The listing builds one solid part. Answer for the finished solid, in the listing's coordinates (mm). A direction names the side the tool comes from. Give positions to 0.01 mm unless a question says otherwise; leave off trailing zeros. Write each loop counter-clockwise with the first axis right and the second up, starting at its lowest first coordinate (ties: lowest second). Pieces come first, ordered by that corner, then holes. Notation, with made-up numbers: (-13, -0.5) - (40, -0.5) arc R18 cw to (40, 24.5) - close; hole circle Ø11 at (22, -3.5). An arc over 180 degrees is marked (long way). One line per item, written item: value. Start each with the question number.
from build123d import *

# Parameters (mm, degrees)
SKETCH_1_W      = 50
SKETCH_1_H      = 14
SKETCH_1_R      = 3
EXTRUDE_1_DEPTH = 5
SKETCH_2_W      = 35
SKETCH_2_H      = 14
EXTRUDE_2_DEPTH = 15
SKETCH_3_W      = 35
SKETCH_3_H      = 5
EXTRUDE_3_DEPTH = 8
SKETCH_4_W      = 12
SKETCH_4_H      = 4
SKETCH_4_W_2    = 6
EXTRUDE_4_DEPTH = 4
FILLET_1_R      = 2


with BuildPart() as part:
    # Эскиз1 → Бобышка-Вытянуть1 (new body)
    with BuildSketch(Plane(origin=(0, 0, 0), x_dir=(1, 0, 0), z_dir=(0, 1, 0))):
        with Locations((-18, 0)):
            Rectangle(SKETCH_1_W, SKETCH_1_H)
        with Locations(Location((0, 0, 0), (0, 0, 270))):
            Circle(SKETCH_1_R, mode=Mode.SUBTRACT)
    extrude(amount=EXTRUDE_1_DEPTH)

    # Эскиз2 → Бобышка-Вытянуть2 (add)
    with BuildSketch(Plane(origin=(0, 5, 0), x_dir=(1, 0, 0), z_dir=(0, 1, 0))):
        with Locations((-25.5, 0)):
            Rectangle(SKETCH_2_W, SKETCH_2_H)
    extrude(amount=EXTRUDE_2_DEPTH)

    # Эскиз3 → Бобышка-Вытянуть3 (add)
    with BuildSketch(Plane(origin=(0, 20, 0), x_dir=(1, 0, 0), z_dir=(0, 1, 0))):
        with Locations((-25.5, -4.5)):
            Rectangle(SKETCH_3_W, SKETCH_3_H)
        with Locations((-25.5, 4.5)):
            Rectangle(SKETCH_3_W, SKETCH_3_H)
    extrude(amount=EXTRUDE_3_DEPTH)

    # Эскиз4 → Бобышка-Вытянуть4 (add)
    with BuildSketch(Plane(origin=(0, 20, 0), x_dir=(1, 0, 0), z_dir=(0, 1, 0))):
        with Locations((-49, 0)):
            Rectangle(SKETCH_4_W, SKETCH_4_H)
        with Locations((-5, 0)):
            Rectangle(SKETCH_4_W_2, SKETCH_4_H)
    extrude(amount=-EXTRUDE_4_DEPTH)

    # Скругление1
    fillet_1_edges = [part.edges().sort_by_distance(p)[0] for p in [
        (-25.5, 28, 7),
        (-25.5, 28, 2),
        (-25.5, 28, -7),
        (-25.5, 28, -2),
    ]]
    fillet(fillet_1_edges, radius=FILLET_1_R)


solid = part.part
Item 1: Each of these flat-tipped pins is pushed along its axis until it touches: pin 1 Ø2 at (x, z) = (-47.5, 0) entering from -Y; pin 2 Ø1.5 at (x, z) = (-20.5, -2.5) entering from +Y; pin 3 Ø3 at (x, y) = (-50, 17.5) entering from +Z; pin 4 Ø4.5 at (x, y) = (-6, 18.5) entering from +Z. Where does it stop, or does it pass through?
Item 2: Straight lines are drawn through the part: line 1 along X through (y, z) = (2.65, 0); line 2 along X through (y, z) = (8, 5); line 3 along Y through (x, z) = (-27, 1.5). For each, find the intervals that lie inside material, in ascending order.
Item 3: Find section D-D on x = -24. Determine the outline of the cut face in (y, z).
Item 4: Find section C-C on z = 0. Determine the outline of the cut face in (x, y).
Item 5: The mould has two halves that part along Y. Classify faces 4 (the flat face through (-5, 16, 0)), 5 (the flat face through (-5, 18, -2)), 6 (the flat face through (-29, 20, 0)): +Y half, -Y half, draft (parallel to the pull), parting line (faces both ways), or undercut.
Item 6: Find section A-A on x = 0. Determine the outline of the cut face in (y, z), plus the area to 3 significant figures.
Item 7: Find section B-B on y = 23.25. Determine the outline of the cut face in (x, z).
Item 8: For faces 1 (the flat face through (-26, 23, -2)), 2 (the flat face through (-49, 18, -2)), 3 (the flat face through (-49, 16, 0)), determine the directions among +Z, -Z, +X, -X, +Y, -Y from which every point of the face is accessible in a straight line to the end or side of a thin tool.
Values:
1. pin 1: y = 16
1. pin 2: y = 27.85
1. pin 3: z = 2
1. pin 4: z = 7
2. line 1: -43 to -3, 3 to 7
2. line 2: -43 to -8
2. line 3: 0 to 20
3. outline: (0, -7) - (26, -7) arc R2 ccw to (28, -5) - (28, -4) arc R2 ccw to (26, -2) - (20, -2) - (20, 2) - (26, 2) arc R2 ccw to (28, 4) - (28, 5) arc R2 ccw to (26, 7) - (0, 7) - close
4. outline: (-55, 16) - (-43, 16) - (-43, 0) - (-3, 0) - (-3, 5) - (-8, 5) - (-8, 16) - (-2, 16) - (-2, 20) - (-55, 20) - close; (3, 0) - (7, 0) - (7, 5) - (3, 5) - close
5. face 4: undercut
5. face 5: draft
5. face 6: +Y half
6. outline: (0, -7) - (5, -7) - (5, -3) - (0, -3) - close; (0, 3) - (5, 3) - (5, 7) - (0, 7) - close
6. area: 40.0 mm^2
7. outline: (-43, -7) - (-8, -7) - (-8, -2) - (-43, -2) - close; (-43, 2) - (-8, 2) - (-8, 7) - (-43, 7) - close
8. face 1: +X, -X, +Y
8. face 2: -Z, -X, +Y, -Y
8. face 3: +Z, -Z, -X, -Y
